from build123d import *

# Parameters (mm, degrees)
CHAMFER1_SIZE     = 0.635
CIRPATTERN2_COUNT = 3
FILLET2_R         = 0.9652


with BuildPart() as part:
    # Sketch1 → Revolve1 (revolve)
    with BuildSketch(Plane.XY, mode=Mode.PRIVATE) as revolve1_sk:
        Polygon((0, 0), (0, 6.35), (1.984375, 6.35), (1.984375, 3.175), (12.7, 3.175), (12.7, 0), align=None)
    revolve(revolve1_sk.sketch.rotate(Axis((0, 0, 0), (1, 0, 0)), 90), axis=Axis((0, 0, 0), (1, 0, 0)))

    # Chamfer1
    chamfer1_edges = [part.edges().sort_by_distance(p)[0] for p in [
        (12.7, 0, -3.175),
    ]]
    chamfer(chamfer1_edges, length=CHAMFER1_SIZE)

    # Sketch3 → Revolve3 (revolve)
    with BuildSketch(Plane.XY):
        with BuildLine():
            Line((0, 4.7625), (-0.9652, 4.7625))
            ThreePointArc((-0.9652, 4.7625), (-0.694208674, 5.535036939), (0, 5.969))
            Line((0, 5.969), (0, 4.7625))
        make_face()
    revolve3 = revolve(axis=Axis((1.984375, 4.7625, 0), (-1, 0, 0)))

    # CirPattern2: Revolve3 ×3 about axis
    cirpattern2_axis = Axis((0, 0, 0), (1, 0, 0))
    for i in range(1, CIRPATTERN2_COUNT):
        add(revolve3.rotate(cirpattern2_axis, i * 360 / CIRPATTERN2_COUNT))

    # Fillet2
    fillet2_edges = [part.edges().sort_by_distance(p)[0] for p in [
        (1.984375, 0, -3.175),
        (1.984375, 0, -6.35),
    ]]
    fillet(fillet2_edges, radius=FILLET2_R)


solid = part.part
Input: part model. Units: mm. Frame: model coordinates. Round coordinates to 2 decimals unless told otherwise and drop trailing zeros. Order: outer loops, then holes, each group sorted by start corner. A loop starts at its lowest first (then second) coordinate and runs counter-clockwise, first axis right, second up.
1. Cut plane D-D, the plane x = 1.75. Output: boundary loops of the cut face in (y, z).
The answers:
outline: circle Ø12.03 at (0, 0)
2. Pin query (flat end, axial travel): P1, Ø4, axis at x = 11, z = 1.5, coming from the +Y side (3 decimals); P2, Ø1.5, axis at y = 3, z = -2, coming from the +X side; P3, Ø4, axis at x = 7, y = 1.5, coming from the -Z side (3 decimals). Return the tip coordinate at first contact, or that it passes through.
The answers:
P1: stops at y = 3.175
P2: stops at x = 12.38
P3: stops at z = -3.175
3. Cut plane A-A, the plane y = 0. Output: boundary loops of the cut face in (x, z) (3 decimals).
The answers:
outline: (0, -6.35) - (1.019, -6.35) arc R0.965 ccw to (1.984, -5.385) - (1.984, -4.14) arc R0.965 cw to (2.95, -3.175) - (12.065, -3.175) - (12.7, -2.54) - (12.7, 2.54) - (12.065, 3.175) - (2.95, 3.175) arc R0.965 cw to (1.984, 4.14) - (1.984, 5.385) arc R0.965 ccw to (1.019, 6.35) - (0, 6.35) - close
4. Mould query, pull axis Z, two halves, no side actions, for faces 1 (the face through (0, 0, 0)), 2 (the face through (1.984, 4, 2)), 3 (the face through (7.57, 1.93, -2.52)). Classes: released by +Z, released by -Z, zero draft, split by the parting line, or undercut.
The answers:
face 1: undercut
face 2: zero draft
face 3: split by the parting line
5. Material intervals for line 1 (X direction, y = -2, z = 0.25); line 2 (X direction, y = 4, z = -2.75); line 3 (Y direction, x = 9.25, z = 0.75), sorted ascending.
The answers:
line 1: x = 0 to 12.7
line 2: x = 0 to 1.98
line 3: y = -3.09 to 3.09
6. Cut plane C-C, the plane x = 6.75. Output: boundary loops of the cut face in (y, z) (3 decimals), then the cut area to 3 significant figures.
The answers:
outline: circle Ø6.35 at (0, 0)
area: 31.7 mm2
